Autodesk Inventor part; units mm, degrees
ref_plane "YZ Plane" through (0, 0, 0) normal (1, 0, 0) x (0, 1, 0)
ref_plane "XZ Plane" through (0, 0, 0) normal (0, 1, 0) x (-1, 0, 0)
ref_plane "XY Plane" through (0, 0, 0) normal (0, 0, 1) x (1, 0, 0)
sketch "Sketch2" plane through (0, 0, 0) normal (0, 1, 0) x (-1, 0, 0)
  line L0 (0, 0) -> (-59, 0)
  line L1 (-59, 0) -> (-59, 78)
  line L2 (-59, 78) -> (0, 78)
  line L3 (0, 78) -> (0, 0)
  dimension "d0" = 59
  dimension "d1" = 78
extrude "Extrusion1" add sketch "Sketch2" along normal blind 25
shell "Shell1" thickness 3 removed faces 1 at (39.3333, 25, 52)
sketch "Sketch4" plane through (59, 0, 0) normal (0, 0, -1) x (-1, 0, 0)
  point P0 (59, 0)
sketch "Sketch5" plane through (3, 3, 3) normal (0, 0, 1) x (1, 0, 0)
  line L0 (0, 0) -> (0, 22)
  line L1 (0, 22) -> (53, 22)
  line L2 (0, 0) -> (53, 0)
  line L3 (53, 0) -> (53, 22)
  line L4 (53, 22) -> (0, 22)
  line L5 (0, 22) -> (0, 0)
  point P0 (-3, -3)
extrude "Extrusion3" cut sketch "Sketch5" against normal blind 10
sketch "Sketch6" plane through (0, 0, 0) normal (-1, 0, 0) x (0, 0, 1)
  line L0 (4.5, 21.3) -> (30.5, 21.3)
  line L1 (30.5, 21.3) -> (30.5, 17.5)
  line L2 (30.5, 17.5) -> (4.5, 17.5)
  line L3 (4.5, 17.5) -> (4.5, 21.3)
  line L4 (0, 0) -> (0, 25)
  line L5 (0, 0) -> (78, 0)
  dimension "d19" = 26
  dimension "d20" = 3.8
  dimension "d21" = 4.5
  dimension "d22" = 17.5
sketch "Sketch7" plane through (59, 0, 78) normal (1, 0, 0) x (0, 0, -1)
  line L0 (0, 0) -> (78, 0)
  line L1 (0, 25) -> (78, 25)
  line L2 (78, 25) -> (78, 0)
  line L3 (78, 0) -> (0, 0)
  line L4 (0, 0) -> (0, 25)
extrude "Extrusion5" add sketch "Sketch7" along normal blind 3
extrude "Extrusion6" cut sketch "Sketch6" against normal through all
sketch "Sketch8" plane through (0, 0, 0) normal (-1, 0, 0) x (0, 0, 1)
  circle A0 centre (50, 19.5) radius 2.5
  point P0 (0, 0)
  dimension "d29" = 5
extrude "Extrusion7" cut sketch "Sketch8" against normal through all
properties part number "arduino box v06"
CAD build for the part. Positions are in the model's coordinates, mm. A direction names the side the tool comes from. Give positions to 0.01 mm unless a question says otherwise; leave off trailing zeros. Order: outer loops, then holes, each group sorted by start corner. A loop starts at its lowest first (then second) coordinate and runs counter-clockwise, first axis right, second up. Notation, with made-up numbers: (-18.5, 57) - (35.5, 57) arc R11 cw to (35.5, 72) - close; hole circle Ø11 at (-39.5, 8). An arc over 180 degrees is marked (long way). Answer in a Markdown table with one row per item.
1. Saw through at C-C, the plane z = 56. Give the cut face in (x, y).
Data:
| item | result |
|---|---|
| outline | (0, 0) - (62, 0) - (62, 25) - (56, 25) - (56, 3) - (3, 3) - (3, 25) - (0, 25) - close |
2. Saw through at A-A, the plane y = 19.5. Give the cut face in (x, z).
Data:
| item | result |
|---|---|
| outline | (0, 0) - (3, 0) - (3, 4.5) - (0, 4.5) - close; (0, 30.5) - (3, 30.5) - (3, 47.5) - (0, 47.5) - close; (0, 52.5) - (3, 52.5) - (3, 75) - (56, 75) - (56, 52.5) - (62, 52.5) - (62, 78) - (0, 78) - close; (56, 0) - (62, 0) - (62, 4.5) - (56, 4.5) - close; (56, 30.5) - (62, 30.5) - (62, 47.5) - (56, 47.5) - close |
3. Probe probe 1 along Y at (x, z) = (1.2, 50); probe 2 along X at (y, z) = (4.5, 14); probe 3 along Y at (x, z) = (5, 36.5). List the from-to ranges inside material, lowest first. Write a range as [from, to].
Data:
| item | result |
|---|---|
| probe 1 | y = [0, 17], [22, 25] |
| probe 2 | x = [0, 3], [56, 62] |
| probe 3 | y = [0, 3] |
4. Saw through at B-B, the plane z = 28.5. Give the cut face in (x, y).
Data:
| item | result |
|---|---|
| outline | (0, 0) - (62, 0) - (62, 17.5) - (56, 17.5) - (56, 3) - (3, 3) - (3, 17.5) - (0, 17.5) - close; (0, 21.3) - (3, 21.3) - (3, 25) - (0, 25) - close; (56, 21.3) - (62, 21.3) - (62, 25) - (56, 25) - close |
5. Pull direction Y, two halves, no side cores. Call faces 4 (the flat face through (59, 21.3, 17)), 5 (the flat face through (3, 14, 38)), 6 (the flat face through (58, 25, 45)): pulls with the +Y half, pulls with the -Y half, needs draft (parallel to the pull), parting line crosses it, or undercut.
Data:
| item | result |
|---|---|
| face 4 | undercut |
| face 5 | needs draft |
| face 6 | pulls with the +Y half |
6. Tool access for faces 1 (the flat face through (59, 17.5, 18)), 2 (the flat face through (31, 0, 40)), 3 (the flat face through (29, 3, 38)): list every direction of +Z, -Z, +X, -X, +Y, -Y with a clear straight run to the whole face (end or side of a thin tool).
Data:
| item | result |
|---|---|
| face 1 | +X, -X |
| face 2 | +Z, -Z, +X, -X, -Y |
| face 3 | -Z, +Y |
7. Flat gauge pins, fed straight in: pin 1 (1 mm diameter, centred on x = 31, y = 10.5, fed in from -Z); pin 2 (1 mm diameter, centred on x = 51, z = 24, fed in from +Y). Where does each tip first touch, or does it go through?
Data:
| item | result |
|---|---|
| pin 1 | stops at z = 75 |
| pin 2 | stops at y = 3 |
8. Saw through at D-D, the plane x = 42. Give the cut face in (y, z), plus the area to 3 significant figures.
Data:
| item | result |
|---|---|
| outline | (0, 0) - (3, 0) - (3, 75) - (25, 75) - (25, 78) - (0, 78) - close |
| area | 300 mm² |
